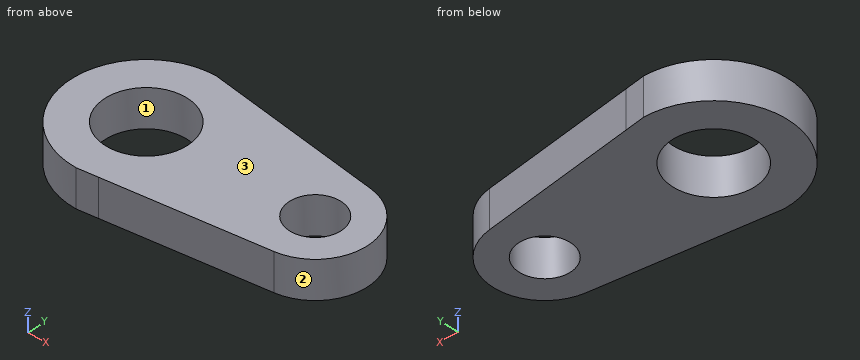
```python
from build123d import *

# Parameters (mm, degrees)
F1_DEPTH = 4
F2_R     = 4.4
F2_R_2   = 2.75
F3_DEPTH = 4


with BuildPart() as f1:
    # F0 (on Top) → F1 (new body)
    with BuildSketch(Plane.XY):
        with BuildLine():
            Line((28.54154, 13.500238), (12.118604, 15.714371))
            Line((12.118604, 15.714371), (10, 16))
            ThreePointArc((10, 16), (2, 8), (10, 0))
            Line((10, 0), (12.118604, 0.285629))
            Line((12.118604, 0.285629), (28.54154, 2.499762))
            ThreePointArc((28.54154, 2.499762), (33.35, 8), (28.54154, 13.500238))
        make_face()
    extrude(amount=F1_DEPTH)

    # F2 (on face) → F3 (cut, through all)
    with BuildSketch(Plane.XY.offset(4)):
        with Locations((10, 8)):
            Circle(F2_R)
        with Locations((27.8, 8)):
            Circle(F2_R_2)
    extrude(amount=-F3_DEPTH, mode=Mode.SUBTRACT)


solid = f1.part
```
Input: part model. Units: mm. Frame: model coordinates. Face numbers are marked on the shaded views. Give positions to 0.01 mm unless a question says otherwise; leave off trailing zeros. Order: outer loops, then holes, each group sorted by start corner. A loop starts at its lowest first (then second) coordinate and runs counter-clockwise, first axis right, second up. Notation, with made-up numbers: M 84.5,21.5 L 112.5,21.5 A13 ccw 112.5,41.5 Z; hole C 5,18 d5. An arc over 180 degrees is marked long. One line per question, with ' | ' between items. Start each with the question number.
1. Section query C-C (x = 30). Return the cut outline in (y, z), and give its area (3 significant figures).
2. Section query D-D (x = 6.5). Return the cut outline in (y, z), and give its area (3 significant figures).
3. Material intervals for probe 1 along Y at (x, z) = (10, 2.6); probe 2 along Y at (x, z) = (7.5, 2.1); probe 3 along X at (y, z) = (7.25, 0.2), sorted ascending. Write a range as [from, to].
4. Pull-direction query (Y, two-part tool) for the marked faces 1, 2 and 3; classes: released by +Y, released by -Y, zero draft, split by the parting line, or undercut.
5. Section query A-A (y = 8). Return the cut outline in (x, z), and give its area (3 significant figures).
6. First-contact query: pin 1 Ø2 at (x, z) = (16.5, 3.5) entering from +Y; pin 2 Ø1.5 at (x, z) = (19, 1) entering from +Y; pin 3 Ø1.5 at (x, z) = (24, 2.5) entering from +Y. Flat tips, straight axial feed; report the tip coordinate or a pass-through.
7. Section query B-B (z = 1.5). Return the cut outline in (x, y), and give its area (3 significant figures).
Here are the results:
1) outline: M 2.9,0 L 6.35,0 L 6.35,4 L 2.9,4 Z; M 9.65,0 L 13.1,0 L 13.1,4 L 9.65,4 Z | area: 27.6 mm²
2) outline: M 0.81,0 L 5.33,0 L 5.33,4 L 0.81,4 Z; M 10.67,0 L 15.19,0 L 15.19,4 L 10.67,4 Z | area: 36.2 mm²
3) probe 1: [0, 3.6], [12.4, 16] | probe 2: [0.4, 4.38], [11.62, 15.6] | probe 3: [2.04, 5.66], [14.34, 25.15], [30.45, 33.3]
4) face 1: undercut | face 2: split by the parting line | face 3: zero draft
5) outline: M 2,0 L 5.6,0 L 5.6,4 L 2,4 Z; M 14.4,0 L 25.05,0 L 25.05,4 L 14.4,4 Z; M 30.55,0 L 33.35,0 L 33.35,4 L 30.55,4 Z | area: 68.2 mm²
6) pin 1: y = 15.26 | pin 2: y = 14.89 | pin 3: y = 14.21
7) outline: M 10,0 L 12.12,0.29 L 28.54,2.5 A5.55 ccw 28.54,13.5 L 12.12,15.71 L 10,16 A8 ccw Z; hole C 10,8 d8.8; hole C 27.8,8 d5.5 | area: 306 mm²
